The listing builds one solid part. Answer for the finished solid, in the listing's coordinates (mm). Give positions to 0.01 mm unless a question says otherwise; leave off trailing zeros. Write each loop counter-clockwise with the first axis right and the second up, starting at its lowest first coordinate (ties: lowest second). Pieces come first, ordered by that corner, then holes. Notation, with made-up numbers: (-9, 51) -> (3, 51) arc R22 ccw to (3, 67) -> close; hole circle Ø7 at (44, -33). An arc over 180 degrees is marked (long way). Put each result on its own line as item: value. Start each with the question number.
1) For a pull along X with two mould halves and no side action, classify faces 1 (the flat face through (-6, -2, 5)), 2 (the conical face through (-2.654, 0.589, 1.719)), 3 (the cylindrical face through (11.923, -3.755, 2.472)), 4 (the cylindrical face through (2.44, 0.54, 0.74)) as released by +X, released by -X, zero draft, split by the parting line, or undercut.
2) Find the intervals of material crossed by line 1 along Y through (x, z) = (0, 0.7); line 2 along X through (y, z) = (-3.5, 1.9); line 3 along Y through (x, z) = (-2.75, 4.75), in increasing order. Write a range as from..to.
3) A cutting plane is placed at C-C (z = 3.25). Write down the section's boundary in (x, y).
4) A flat-ended cylindrical pin translates along its axis: pin 1 Ø3 at (y, z) = (-7, 4) entering from -X (3 decimals). Find the tip coordinate at first contact, or state that the pin passes through.
5) A cutting plane is placed at A-A (y = 0). Write down the section's boundary in (x, z), then the cut area to 4 significant figures.
Autodesk Inventor part; units mm, degrees
ref_plane "YZ Plane" through (0, 0, 0) normal (1, 0, 0) x (0, 1, 0)
ref_plane "XZ Plane" through (0, 0, 0) normal (0, 1, 0) x (-1, 0, 0)
ref_plane "XY Plane" through (0, 0, 0) normal (0, 0, 1) x (1, 0, 0)
sketch "Skizze1" plane through (0, 0, 0) normal (0, 0, 1) x (1, 0, 0)
  circle A0 centre (0, 0) radius 12.5
  dimension "d0" = 25
extrude "Extrusion1" add sketch "Skizze1" along normal blind 5
chamfer "Fasen1" distance 0.5 angle 45 2 edges at (-12.5, 0, 0) (-12.5, 0, 5)
sketch "Skizze2" plane through (0, 0, 5) normal (0, 0, 1) x (1, 0, 0)
  circle A0 centre (0, 0) radius 12
hole "Bohrung1" at (0, 0, 5) direction (0, 0, -1) diameter 5 end through all countersink diameter 12 countersink angle 90
properties part number "Magnet"
Reply:
1. face 1: zero draft
1. face 2: undercut
1. face 3: split by the parting line
1. face 4: undercut
2. line 1: y = -12.5..-2.5, 2.5..12.5
2. line 2: x = -12..12
2. line 3: y = -11.94..-5.05, 5.05..11.94
3. outline: circle Ø25 at (0, 0); hole circle Ø8.5 at (0, 0)
4. pin 1: stops at x = -11.225
5. outline: (-12.5, 0.5) -> (-12, 0) -> (-2.5, 0) -> (-2.5, 1.5) -> (-6, 5) -> (-12, 5) -> (-12.5, 4.5) -> close; (2.5, 0) -> (12, 0) -> (12.5, 0.5) -> (12.5, 4.5) -> (12, 5) -> (6, 5) -> (2.5, 1.5) -> close
5. area: 87.25 mm2
